Input: part model. Units: mm. Frame: model coordinates. A direction names the side the tool comes from. Round coordinates to 2 decimals unless told otherwise and drop trailing zeros. Write each loop counter-clockwise with the first axis right and the second up, starting at its lowest first coordinate (ties: lowest second). Pieces come first, ordered by that corner, then holes. Notation, with made-up numbers: (38.5, 83.5) -> (53.5, 83.5) arc R18 ccw to (53.5, 115.5) -> close; hole circle Ø10 at (60.25, -18). An arc over 180 degrees is marked (long way). Write item = value, one per line.
```python
from build123d import *

# Parameters (mm, degrees)
BOSS_EXTRUDE1_DEPTH = 234
CUT_EXTRUDE1_DEPTH  = 78
BOSS_EXTRUDE2_DEPTH = 33
CUT_EXTRUDE2_DEPTH  = 13
SKETCH6_W           = 33
SKETCH6_H           = 84.469943203
CUT_EXTRUDE3_DEPTH  = 19
CHAMFER2_SIZE       = 1.749773271
CHAMFER2_SIZE_2     = 20


with BuildPart() as part:
    # Sketch1 → Boss-Extrude1 (new body)
    with BuildSketch(Plane(origin=(0, 0, 0), x_dir=(0, 0, -1), z_dir=(1, 0, 0))):
        with BuildLine():
            Line((0, 0), (-13, 0))
            Line((-13, 0), (-84, 40.991869112))
            Line((-84, 40.991869112), (-84, 84))
            ThreePointArc((-84, 84), (-59.39696962, 143.39696962), (0, 168))
            Line((0, 168), (0, 112.575))
            ThreePointArc((0, 112.575), (-28.575, 84), (0, 55.425))
            Line((0, 55.425), (0, 0))
        make_face()
    extrude(amount=BOSS_EXTRUDE1_DEPTH)

    # Sketch2 → Cut-Extrude1 (cut)
    with BuildSketch(Plane(origin=(234, 0, 0), x_dir=(0, 0, -1), z_dir=(1, 0, 0))):
        with BuildLine():
            Line((0, 128.45), (0, 39.55))
            ThreePointArc((0, 39.55), (-44.45, 84), (0, 128.45))
        make_face()
    extrude(amount=-CUT_EXTRUDE1_DEPTH, mode=Mode.SUBTRACT)

    # Sketch3 → Boss-Extrude2 (add)
    with BuildSketch(Plane(origin=(234, 0, 0), x_dir=(0, 0, -1), z_dir=(1, 0, 0))):
        with BuildLine():
            Line((-83.014649379, 96.828405531), (-65.430668922, 83.090294344))
            Line((-65.430668922, 83.090294344), (-14.946427946, 147.707176139))
            Line((-14.946427946, 147.707176139), (-32.530408402, 161.445287327))
            ThreePointArc((-32.530408402, 161.445287327), (-66.192903303, 135.715563927), (-83.014649379, 96.828405531))
        make_face()
    extrude(amount=BOSS_EXTRUDE2_DEPTH)

    # Sketch4 → Cut-Extrude2 (cut)
    with BuildSketch(Plane(origin=(0, 0, 0), x_dir=(-1, 0, 0), z_dir=(0, 0, -1))):
        with BuildLine():
            Line((0, 15), (-117, 15))
            ThreePointArc((-117, 15), (-128, 26), (-117, 37))
            Line((-117, 37), (0, 37))
            ThreePointArc((0, 37), (11, 26), (0, 15))
        make_face()
    extrude(amount=-CUT_EXTRUDE2_DEPTH, mode=Mode.SUBTRACT)

    # Sketch6 → Cut-Extrude3 (cut)
    with BuildSketch(Plane(origin=(0, 0, 0), x_dir=(-1, 0, 0), z_dir=(0, 0, -1))):
        with Locations((-54.5, 125.765028398)):
            Rectangle(SKETCH6_W, SKETCH6_H)
    extrude(amount=-CUT_EXTRUDE3_DEPTH, mode=Mode.SUBTRACT)

    # Chamfer2
    # the kernel refuses this chamfer: 20, 1.749773271 mm, written as the material it adds along each edge
    with BuildSketch(Plane(origin=(38, 53.350481829, 19), x_dir=(0.9159861691531124, 0, 0.4012098427509048), z_dir=(0, 1, 0))) as chamfer2_piece_1_section:
        Polygon((CHAMFER2_SIZE * 0.915986168901, CHAMFER2_SIZE * 0.40120984264), (-CHAMFER2_SIZE_2 * 0.401209842751, CHAMFER2_SIZE_2 * 0.915986169153), (0, 0), align=None)
    chamfer2_piece_1 = extrude(amount=164.465179425, mode=Mode.PRIVATE)
    chamfer2_piece_1 = chamfer2_piece_1 - Plane(origin=(38.476894186, 84, 0), x_dir=(0, 1, 0), z_dir=(-1, 0, 0)) * Cylinder(28.575, 403, mode=Mode.PRIVATE)
    chamfer2_piece_1 = split(chamfer2_piece_1, bisect_by=Plane(origin=(38.476894186, 56.471998141, 0), z_dir=(0, 0, 1)), keep=Keep.TOP, mode=Mode.PRIVATE)
    chamfer2_piece_1 = chamfer2_piece_1 & Plane(origin=(38.476894186, 84, 0), x_dir=(0, 0, 1), z_dir=(-1, 0, 0)) * Cylinder(84, 403, mode=Mode.PRIVATE)
    add(chamfer2_piece_1)
    with BuildSketch(Plane(origin=(71, 217.815661254, 19), x_dir=(0.003352615794032912, 0, -0.9999943799678763), z_dir=(0, -1, 0))) as chamfer2_piece_2_section:
        Polygon((CHAMFER2_SIZE_2 * 0.999994379968, -CHAMFER2_SIZE_2 * 0.00335261579403), (-CHAMFER2_SIZE * 0.00335261579311, -CHAMFER2_SIZE * 0.999994379693), (0, 0), align=None)
    chamfer2_piece_2 = extrude(amount=164.465179425, mode=Mode.PRIVATE)
    chamfer2_piece_2 = chamfer2_piece_2 - Plane(origin=(70.625797468, 84, 0), x_dir=(0, 1, 0), z_dir=(-1, 0, 0)) * Cylinder(28.575, 409, mode=Mode.PRIVATE)
    chamfer2_piece_2 = chamfer2_piece_2 & Plane(origin=(70.625797468, 84, 0), x_dir=(0, 0, 1), z_dir=(-1, 0, 0)) * Cylinder(84, 409, mode=Mode.PRIVATE)
    chamfer2_piece_2 = split(chamfer2_piece_2, bisect_by=Plane(origin=(70.625797468, 138.170488536, 0), z_dir=(0, 0, 1)), keep=Keep.TOP, mode=Mode.PRIVATE)
    add(chamfer2_piece_2)


solid = part.part
```
1) Cut plane B-B (z = 74.5). Return the cut outline in (x, y), and give its area (3 significant figures).
Solutions:
outline = (0, 35.51) -> (234, 35.51) -> (234, 90.18) -> (267, 90.18) -> (267, 122.8) -> (0, 122.8) -> close
area = 21,500 mm^2
2) First-contact query: P1, Ø1.5, axis at x = 49, y = 21, coming from the +Z side; P2, Ø12, axis at x = 46, y = 22.5, coming from the +Z side; P3, Ø5, axis at x = 123, z = 40.5, coming from the -Y side. Flat tips, straight axial feed; report the tip coordinate or a pass-through.
Solutions:
P1 = 50.67
P2 = 62.36
P3 = 14.43
3) Cut plane A-A (x = 134.5). Return the cut outline in (y, z) (3 decimals).
Solutions:
outline = (0, 0) -> (55.425, 0) arc R28.575 cw to (112.575, 0) -> (168, 0) arc R84 ccw to (84, 84) -> (40.992, 84) -> (0, 13) -> close
4) Cut plane D-D (x = 59). Return the cut outline in (y, z) (3 decimals).
Solutions:
outline = (0, 0) -> (15, 0) -> (15, 13) -> (37, 13) -> (37, 0) -> (55.425, 0) arc R28.575 cw to (105.343, 19) -> (165.823, 19) arc R84 ccw to (84, 84) -> (40.992, 84) -> (0, 13) -> close
5) Cut plane C-C (y = 26). Return the cut outline in (x, z).
Solutions:
outline = (0, 13) -> (128, 13) -> (128, 0) -> (234, 0) -> (234, 58.03) -> (0, 58.03) -> close
6) Line query: L1, parallel to Y at x = 76.5, z = 11; L2, parallel to X at y = 50, z = 60.5; L3, parallel to Y at x = 68, z = 6. Output: solid intervals per line, ascending. Write a range as from..to.
Solutions:
L1 = 0..15, 37..57.63, 110.37..167.28
L2 = 0..234
L3 = 0..15, 37..56.06
7) Draft query along X for faces 5 (the face through (128, 26, 6)), 6 (the face through (38.93, 136.23, 9.63)), 7 (the face through (59, 37, 6)), 8 (the face through (70.093, 137.11, 9.367)). Return one class per face: +X half, -X half, draft (parallel to the pull), parting line (faces both ways), or undercut.
Solutions:
face_5 = -X half
face_6 = undercut
face_7 = draft
face_8 = undercut
8) Access query for faces 1 (the face through (63, 26, 13)), 2 (the face through (250.269, 154.48, 23.615)), 3 (the face through (250.27, 90.06, 74.35)), 4 (the face through (195.55, 83.02, 44.44)). Directions: +Z, -Z, +X, -X, +Y, -Y. A direction counts if a zero-diameter tool reaches every point of the face in a straight line with its end or side. Return the directions, or none.
Solutions:
face_1 = -Z, -X
face_2 = -Z, +X, +Y
face_3 = +Z, +X, -Y
face_4 = -Z, +X
